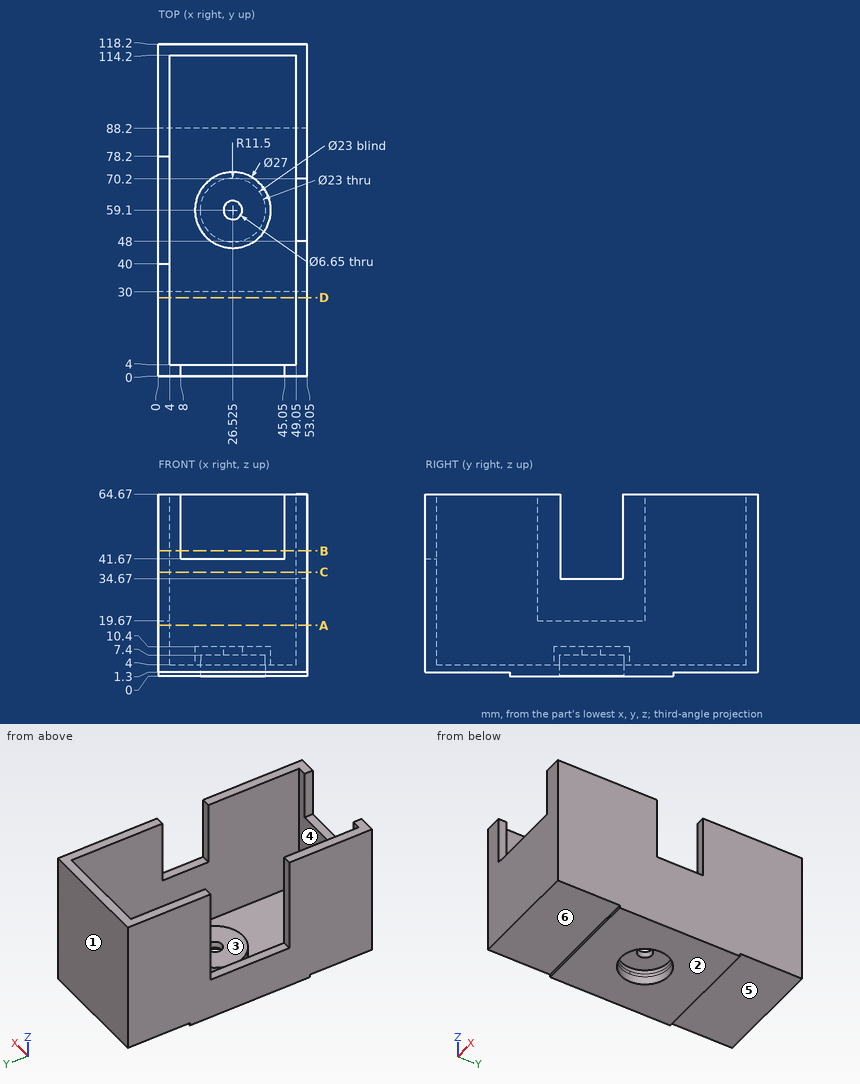
Drawing for the job (mm, zero at the part's lowest x, y, z). A direction names the side the tool comes from. Give positions to 0.01 mm unless a question says otherwise; leave off trailing zeros. Loops run counter-clockwise (first coordinate to the right, second up) from the corner with the lowest first, then second, coordinate; pieces in that order, holes last.
Item 1: Slice it at A-A (z = 18). Write the cut outline in (x, y), plus the area to 3 significant figures.
Check values:
outline: (0, 0) - (53.05, 0) - (53.05, 118.2) - (0, 118.2) - close; hole (4, 4) - (49.05, 4) - (49.05, 114.2) - (4, 114.2) - close
area: 1,310 mm2
Item 2: Slice it at D-D (y = 28). Write the cut outline in (x, z).
Check values:
outline: (0, 1.3) - (53.05, 1.3) - (53.05, 64.67) - (49.05, 64.67) - (49.05, 4) - (4, 4) - (4, 64.67) - (0, 64.67) - close
Item 3: Slice it at C-C (z = 37). Write the cut outline in (x, y).
Check values:
outline: (0, 0) - (53.05, 0) - (53.05, 48) - (49.05, 48) - (49.05, 4) - (4, 4) - (4, 40) - (0, 40) - close; (0, 78.2) - (4, 78.2) - (4, 114.2) - (49.05, 114.2) - (49.05, 70.2) - (53.05, 70.2) - (53.05, 118.2) - (0, 118.2) - close
Item 4: Drop flat-ended pins along their axis: P1, Ø12, axis at y = 71.5, z = 30.5, coming from the -X side; P2, Ø13.5, axis at x = 32, y = 83, coming from the +Z side; P3, Ø8.5, axis at x = 26.525, y = 59.1, coming from the -Z side. Give the stop position or say it passes through.
Check values:
P1: stops at x = 49.05
P2: stops at z = 4
P3: stops at z = 7.4
Item 5: Mould opens along Y. For the marked faces 1, 2 and 3 say: +Y half, -Y half, draft (parallel to the pull), parting line (faces both ways), or undercut.
Check values:
face 1: +Y half
face 2: draft
face 3: undercut
Item 6: Which spindle directions (+Z, -Z, +X, -X, +Y, -Y) get a long thin tool onto all of the face, cutting with end or side? Do the marked faces 4, 5 and 6. Say none if no direction does.
Check values:
face 4: +Z
face 5: -Z, +X, -X, +Y
face 6: -Z, +X, -X, -Y
Item 7: Drill centre lines: line 1 along Y through (x, z) = (49.5, 54); line 2 along X through (y, z) = (19, 19); line 3 along Y through (x, z) = (5, 39). Where is each one in solid material? Low to high.
Check values:
line 1: y = 0 to 48, 70.2 to 118.2
line 2: x = 0 to 4, 49.05 to 53.05
line 3: y = 0 to 4, 114.2 to 118.2
Item 8: Slice it at B-B (z = 44.5). Write the cut outline in (x, y).
Check values:
outline: (0, 0) - (8, 0) - (8, 4) - (4, 4) - (4, 40) - (0, 40) - close; (0, 78.2) - (4, 78.2) - (4, 114.2) - (49.05, 114.2) - (49.05, 70.2) - (53.05, 70.2) - (53.05, 118.2) - (0, 118.2) - close; (45.05, 0) - (53.05, 0) - (53.05, 48) - (49.05, 48) - (49.05, 4) - (45.05, 4) - close
